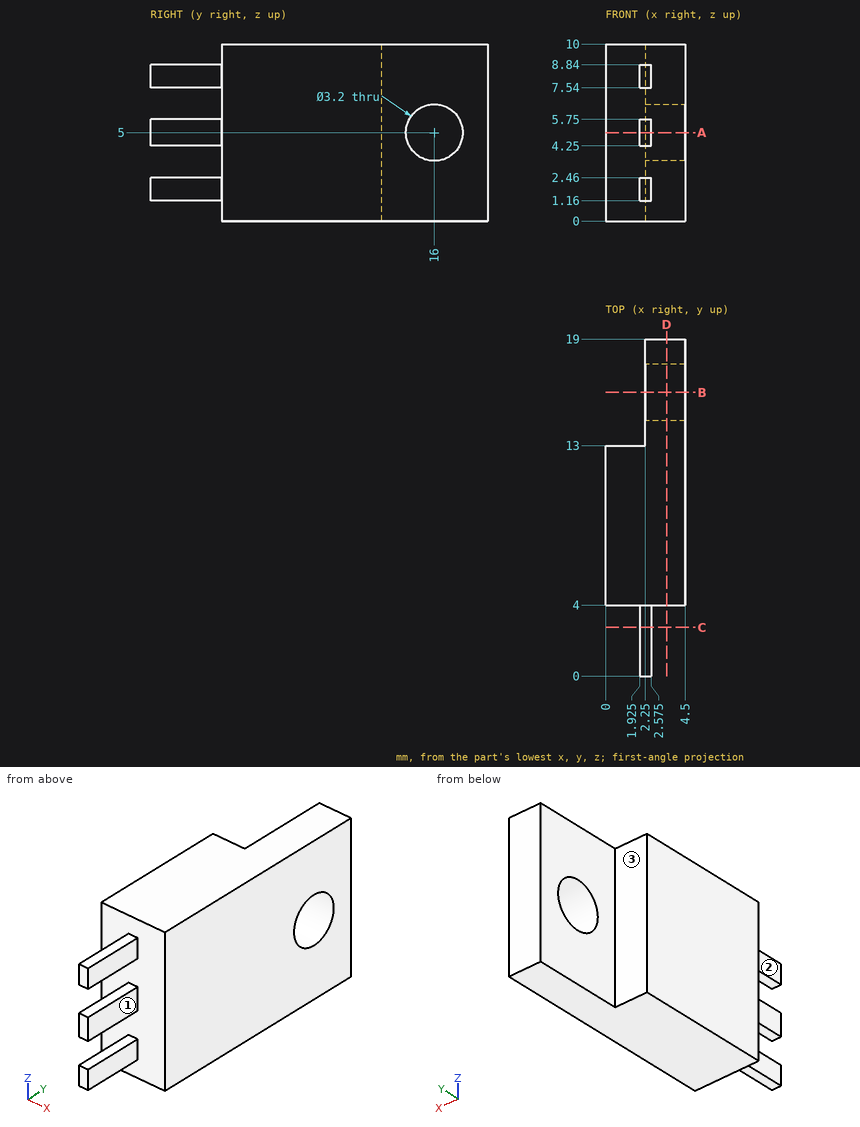
Verification items for this drawing (mm, ordinates from the low corner). A direction names the side the tool comes from. Round coordinates to 2 decimals unless told otherwise and drop trailing zeros. Write each loop counter-clockwise with the first axis right and the second up, starting at its lowest first coordinate (ties: lowest second). Pieces come first, ordered by that corner, then holes. Notation, with made-up numbers: (19, 24) - (52, 24) arc R17 cw to (52, 46) - close; hole circle Ø9 at (-16.5, 55). An arc over 180 degrees is marked (long way). One line per item, written item: value.
1. Cross-section at D-D on x = 3.45. Record the boundary of the cut face in (y, z), and give its area (3 significant figures).
The answers:
outline: (4, 0) - (19, 0) - (19, 10) - (4, 10) - close; hole circle Ø3.2 at (16, 5)
area: 142 mm^2
2. Cross-section at B-B on y = 16. Record the boundary of the cut face in (x, z).
The answers:
outline: (2.25, 0) - (4.5, 0) - (4.5, 3.4) - (2.25, 3.4) - close; (2.25, 6.6) - (4.5, 6.6) - (4.5, 10) - (2.25, 10) - close
3. Cross-section at C-C on y = 2.75. Record the boundary of the cut face in (x, z) (3 decimals), and give its area (4 significant figures).
The answers:
outline: (1.925, 1.16) - (2.575, 1.16) - (2.575, 2.46) - (1.925, 2.46) - close; (1.925, 4.25) - (2.575, 4.25) - (2.575, 5.75) - (1.925, 5.75) - close; (1.925, 7.54) - (2.575, 7.54) - (2.575, 8.84) - (1.925, 8.84) - close
area: 2.665 mm^2
4. Set-up check for the marked faces 1, 2 and 3: record each of +Z, -Z, +X, -X, +Y, -Y from which the full face is reachable in a straight line by a thin tool's end or side.
The answers:
face 1: +Z, -Z, +X, -Y
face 2: +Z, -Z, -X, -Y
face 3: +Z, -Z, -X, +Y
5. Depth check by flat-ended pin: pin 1 Ø1.1 at (x, z) = (1.5, 2.5) entering from +Y; pin 2 Ø2 at (x, y) = (4, 15.5) entering from -Z; pin 3 Ø1.4 at (y, z) = (3, 2) entering from -X (3 decimals); pin 4 Ø0.7 at (y, z) = (1, 2) entering from +X (3 decimals). Enter the tip coordinate at first touch or a pass-through.
The answers:
pin 1: stops at y = 13
pin 2: stops at z = 0
pin 3: stops at x = 1.925
pin 4: stops at x = 2.575
6. Cross-section at A-A on z = 5. Record the boundary of the cut face in (x, y) (3 decimals).
The answers:
outline: (0, 4) - (1.925, 4) - (1.925, 0) - (2.575, 0) - (2.575, 4) - (4.5, 4) - (4.5, 14.4) - (2.25, 14.4) - (2.25, 13) - (0, 13) - close; (2.25, 17.6) - (4.5, 17.6) - (4.5, 19) - (2.25, 19) - close
7. Scan lines: L1, parallel to Y at x = 3.1, z = 5; L2, parallel to Y at x = 3.15, z = 9; L3, parallel to X at y = 1.25, z = 5 (3 decimals). Record each from-to range of solid material in increasing order.
The answers:
L1: y = 4 to 14.4, 17.6 to 19
L2: y = 4 to 19
L3: x = 1.925 to 2.575
